Autodesk Inventor part; units mm, degrees
ref_plane "Plano de trabajo1" through (29.6626, 0, -10) normal (0, 0, 1) x (1, 0, 0)
ref_plane "YZ Plane" through (0, 0, 0) normal (1, 0, 0) x (0, 1, 0)
ref_plane "XZ Plane" through (0, 0, 0) normal (0, 1, 0) x (-1, 0, 0)
sketch "Boceto1" plane through (0, 0, 0) normal (0, 1, 0) x (-1, 0, 0)
  line L0 (52.4225, 0) -> (-52.4225, 0)
  line L1 (38.3374, 0) -> (38.3374, -8)
  line L2 (38.3374, -8) -> (-29.6626, -8)
  line L3 (-29.6626, -8) -> (-29.6626, 0)
  line L4 (38.3374, -5) -> (27.3374, -5)
  line L5 (27.3374, -5) -> (27.3374, 0)
  line L6 (33.3374, -8) -> (33.3374, -8.1)
  line L7 (33.3374, -8.1) -> (27.3374, -8.1)
  line L8 (27.3374, -8.1) -> (27.3374, -8)
  arc A0 (-37.6626, 0) -> (-29.6626, -8) centre (-29.6626, 0) ccw
  line L9 (-18.6626, 2) -> (-37.6626, 2)
  line L10 (-37.6626, 2) -> (-37.6626, -2)
  line L11 (-37.6626, -2) -> (-18.6626, -2)
  line L12 (-18.6626, -2) -> (-18.6626, 2)
  point P0 (0, 0)
  point P1 (0, 0)
  point P2 (-29.6626, -10)
  dimension "d0" = 68
  dimension "d1" = 16
  dimension "d2" = 10
  dimension "d3" = 11
  dimension "d4" = 5
  dimension "d5" = 6
  dimension "d6" = 16.2
  dimension "d8" = 8
  dimension "d9" = 19
  dimension "d10" = 4
  dimension "d11" = 10
  dimension "d12" = 38.3374
  dimension "d13" = 14.0851
  dimension "d14" = 68
revolve "Revolución1" add sketch "Boceto1" angle 360 about axis through (-52.4225, 0, 0) along (1, 0, 0) contours L5 L4 L1 L2 L3 L11 L12 L0 | L12 L11 L3 L0 | L3 L11 A0 L0 | L6 L7 L8 L2 | L3 A0 L11
extrude "Extrusión1" cut sketch "Boceto1" along normal through all both and the other way through all contours L12 L11 L3 L0 | L0 L10 L9 L12 | L3 L11 A0 L0 | A0 L11 L10
ref_plane "Plano de trabajo1" through (29.6626, 0, -10) normal (0, 0, 1) x (1, 0, 0)
sketch "Boceto2" plane through (29.6626, 0, -10) normal (0, 0, 1) x (1, 0, 0)
  line L0 (-11, 7.746) -> (0, 7.746)
  line L1 (0, -7.746) -> (0, 7.746)
  line L2 (0, -7.746) -> (-11, -7.746)
  line L3 (-11, -7.746) -> (-11, -7.746)
  line L4 (-11, -7.746) -> (0, -7.746)
  line L5 (0, 7.746) -> (0, -7.746)
  line L6 (0, 7.746) -> (-11, 7.746)
  line L7 (-11, 7.746) -> (-11, 7.746)
  line L8 (-57, -8) -> (-57, 8)
  arc A0 (0, -7.746) -> (0, 7.746) centre (0, 0) ccw
  line L9 (0, -7.746) -> (0, 7.746)
  point P0 (-29.6626, 0)
hole "Agujero1" at (29.6626, 0, -10) direction (0, 0, 1) diameter 5 end through all
properties part number "1 -HUDSON-8-31B-TDR HAND PUMP"
Input: part model. Units: mm. Frame: model coordinates. A direction names the side the tool comes from. Round coordinates to 2 decimals unless told otherwise and drop trailing zeros. Write each loop counter-clockwise with the first axis right and the second up, starting at its lowest first coordinate (ties: lowest second). Pieces come first, ordered by that corner, then holes.
1) Draft query along Y for faces 1 (the flat face through (-27.337, 0, 0)), 2 (the cylindrical face through (-35.8, -7.81, 1.73)), 3 (the flat face through (26, 0, -2)). Return one class per face: pulls with the +Y half, pulls with the -Y half, needs draft (parallel to the pull), parting line crosses it, or undercut.
2) Cut plane D-D (z = -6.5). Return the cut outline in (x, y), then the cut area to 3 significant figures.
3) Contact query for flat-ended pins moving along their axis: P1, Ø1.5, axis at x = 17, z = -2.5, coming from the +Y side; P2, Ø2, axis at y = 2, z = 0.5, coming from the -X side; P3, Ø1, axis at y = 4.5, z = 4, coming from the +X side; P4, Ø5, axis at y = 2.5, z = 1.5, coming from the +X side. Output: stop coordinate, or through.
4) Cut plane C-C (x = 22). Return the cut outline in (y, z), then the cut area to 3 significant figures.
5) Reachability of faces 4 (the cylindrical face through (1.56, -3.06, -7.39)), 5 (the flat face through (18.663, 0, 0)), 6 (the cylindrical face through (-32.76, -4.88, 1.08)) from +Z, -Z, +X, -X, +Y, -Y: full face, straight path, thin tool, end or side. Return the list, or none.
6) Cut plane B-B (z = 0). Return the cut outline in (x, y), then the cut area to 3 significant figures.
7) Cut plane A-A (y = 0). Return the cut outline in (x, z).
8) Ray query, L1, parallel to X at y = -2, z = 4.75; L2, parallel to X at y = -7, z = 1; L3, parallel to Z at x = 4.5, y = 0.5. Return the intervals inside material, ascending.
Geometry says:
1. face 1: undercut
1. face 2: parting line crosses it
1. face 3: needs draft
2. outline: (-38.34, -4.66) - (-33.34, -4.66) - (-33.34, -4.83) - (-27.34, -4.83) - (-27.34, -4.66) - (29.66, -4.66) arc R4.66 ccw to (29.66, 4.66) - (-27.34, 4.66) - (-27.34, 4.83) - (-33.34, 4.83) - (-33.34, 4.66) - (-38.34, 4.66) - close; hole circle Ø5 at (29.66, 0)
2. area: 651 mm2
3. P1: stops at y = 7.81
3. P2: stops at x = -27.34
3. P3: stops at x = 35.45
3. P4: stops at x = 37.41
4. outline: (-7.75, -2) arc R8 ccw to (7.75, -2) - close; (-7.75, 2) - (7.75, 2) arc R8 ccw to start
4. area: 138 mm2
5. face 4: +X
5. face 5: +X, +Y, -Y
5. face 6: -X
6. outline: (-38.34, -8) - (-33.34, -8) - (-33.34, -8.1) - (-27.34, -8.1) - (-27.34, -8) - (18.66, -8) - (18.66, 8) - (-27.34, 8) - (-27.34, 8.1) - (-33.34, 8.1) - (-33.34, 8) - (-38.34, 8) - (-38.34, 5) - (-27.34, 5) - (-27.34, -5) - (-38.34, -5) - close
6. area: 803 mm2
7. outline: (-38.34, -8) - (-33.34, -8) - (-33.34, -8.1) - (-27.34, -8.1) - (-27.34, -8) - (27.16, -8) - (27.16, -2) - (18.66, -2) - (18.66, 2) - (27.16, 2) - (27.16, 8) - (-27.34, 8) - (-27.34, 8.1) - (-33.34, 8.1) - (-33.34, 8) - (-38.34, 8) - (-38.34, 5) - (-27.34, 5) - (-27.34, -5) - (-38.34, -5) - close; (32.16, -7.6) arc R8 ccw to (37.41, -2) - (32.16, -2) - close; (32.16, 2) - (37.41, 2) arc R8 ccw to (32.16, 7.6) - close
8. L1: x = -38.34 to 28.16, 31.16 to 35.78
8. L2: x = -38.34 to 18.66
8. L3: z = -7.98 to 7.98
